Could you check a few things on this model? Use its own coordinates, in mm. A direction names the side the tool comes from. Coordinates: 2 decimals unless noted, no trailing zeros. Order: outer loops, then holes, each group sorted by start corner. A loop starts at its lowest first (then second) coordinate and runs counter-clockwise, first axis right, second up. Notation, with made-up numbers: M 11.25,55 L 56.25,55 A11 ccw 56.25,68 Z; hole C 73,-10.75 d10. An arc over 180 degrees is marked long. Write item = value, one per line. Start each with the question number.
from build123d import *

# Parameters (mm, degrees)
BOSS_EXTRUDE1_DEPTH = 40
SKETCH2_R           = 2.15
SKETCH2_R_2         = 1.5
CUT_EXTRUDE1_DEPTH  = 44.618574025
SKETCH3_R           = 1.5
CUT_EXTRUDE2_DEPTH  = 44.618574025


with BuildPart() as part:
    # Sketch1 → Boss-Extrude1 (new body)
    with BuildSketch(Plane(origin=(0, 0, 0), x_dir=(1, 0, 0), z_dir=(0, 1, 0))):
        Polygon((0, 0), (0, 0.7), (14, 0.7), (14, 9.3), (14.7, 9.3), (14.7, 0), align=None)
    extrude(amount=BOSS_EXTRUDE1_DEPTH)

    # Sketch2 → Cut-Extrude1 (cut, through all)
    with BuildSketch(Plane(origin=(14.7, 0, 0), x_dir=(0, 0, -1), z_dir=(1, 0, 0))):
        with Locations((5.3, 35)):
            Circle(SKETCH2_R)
        with Locations((5.3, 25)):
            Circle(SKETCH2_R)
        with Locations((5.3, 15)):
            Circle(SKETCH2_R_2)
        with Locations((5.3, 5)):
            Circle(SKETCH2_R_2)
    extrude(amount=-CUT_EXTRUDE1_DEPTH, mode=Mode.SUBTRACT)

    # Sketch3 → Cut-Extrude2 (cut, through all)
    with BuildSketch(Plane.XY):
        with Locations((6, 15.001223109)):
            Circle(SKETCH3_R)
        with Locations((6, 5)):
            Circle(SKETCH3_R)
    extrude(amount=-CUT_EXTRUDE2_DEPTH, mode=Mode.SUBTRACT)


solid = part.part
(1) Imagine slicing it at C-C on z = -5.3. List the corners of the cut face in (x, y) for me.
(2) Imagine slicing it at A-A on x = 6. List the corners of the cut face in (y, z) for me, plus the area to 3 significant figures.
(3) Imagine slicing it at D-D on y = 5. List the corners of the cut face in (x, z) for me.
(4) Imagine slicing it at B-B on y = 35. List the corners of the cut face in (x, z) for me.
(5) For faces 1 (the flat face through (7, 20, -0.7)), 2 (the cylindrical face through (14.35, 15.07, -3.8)), which set-ups out of +Z, -Z, +X, -X, +Y, -Y let a thin tool reach every point of the face, with its end or its side?
(6) Please list where these lines run through material, in increasing order: probe 1 along Y at (x, z) = (14.5, -5.3); probe 2 along Y at (x, z) = (6, -0.45); probe 3 along X at (y, z) = (3, -4.5). Write a range as from..to.
(7) Will these pins go through, and if not, where does the flat tip stop? P1, Ø4, axis at y = 30.5, z = -1, coming from the -X side; P2, Ø1.5, axis at x = 11.5, y = 24, coming from the -Z side; P3, Ø4, axis at y = 12.5, z = -4, coming from the -X side.
(8) Thinking about a two-plate mould opening in X: for faces 3 (the cylindrical face through (4.8, 4.1, -0.3)), 4 (the flat face through (7, 20, 0)), 5 (the flat face through (14, 20, -5)), which applies, released by +X, released by -X, zero draft, split by the parting line, or undercut?
Response:
q1.outline = M 14,0 L 14.7,0 L 14.7,3.5 L 14,3.5 Z; M 14,6.5 L 14.7,6.5 L 14.7,13.5 L 14,13.5 Z; M 14,16.5 L 14.7,16.5 L 14.7,22.85 L 14,22.85 Z; M 14,27.15 L 14.7,27.15 L 14.7,32.85 L 14,32.85 Z; M 14,37.15 L 14.7,37.15 L 14.7,40 L 14,40 Z
q2.outline = M 0,-0.7 L 3.5,-0.7 L 3.5,0 L 0,0 Z; M 6.5,-0.7 L 13.5,-0.7 L 13.5,0 L 6.5,0 Z; M 16.5,-0.7 L 40,-0.7 L 40,0 L 16.5,0 Z
q2.area = 23.8 mm2
q3.outline = M 0,-0.7 L 4.5,-0.7 L 4.5,0 L 0,0 Z; M 7.5,-0.7 L 14,-0.7 L 14,-3.8 L 14.7,-3.8 L 14.7,0 L 7.5,0 Z; M 14,-9.3 L 14.7,-9.3 L 14.7,-6.8 L 14,-6.8 Z
q4.outline = M 0,-0.7 L 14,-0.7 L 14,-3.15 L 14.7,-3.15 L 14.7,0 L 0,0 Z; M 14,-9.3 L 14.7,-9.3 L 14.7,-7.45 L 14,-7.45 Z
q5.face_1 = -Z, -X, +Y, -Y
q5.face_2 = +X, -X
q6.probe_1 = 0..3.5, 6.5..13.5, 16.5..22.85, 27.15..32.85, 37.15..40
q6.probe_2 = 0..3.5, 6.5..13.5, 16.5..40
q6.probe_3 = 14..14.7
q7.P1 = 0
q7.P2 = -0.7
q7.P3 = 14
q8.face_3 = undercut
q8.face_4 = zero draft
q8.face_5 = released by -X
